from build123d import *

# Parameters (mm, degrees)
SKETCH1_R           = 15
SKETCH1_R_2         = 1.5
SKETCH1_R_3         = 4.7
BOSS_EXTRUDE2_DEPTH = 10
SKETCH2_R           = 1.5
CUT_EXTRUDE1_DEPTH  = 35


with BuildPart() as part:
    # Sketch1 → Boss-Extrude2 (new body)
    with BuildSketch(Plane.XY):
        Circle(SKETCH1_R)
        with Locations((0, 10)):
            Circle(SKETCH1_R_2, mode=Mode.SUBTRACT)
        Circle(SKETCH1_R_3, mode=Mode.SUBTRACT)
        with Locations((10, 0)):
            Circle(SKETCH1_R_2, mode=Mode.SUBTRACT)
        with Locations((0, -10)):
            Circle(SKETCH1_R_2, mode=Mode.SUBTRACT)
        with Locations((-10, 0)):
            Circle(SKETCH1_R_2, mode=Mode.SUBTRACT)
    extrude(amount=BOSS_EXTRUDE2_DEPTH)

    # Sketch2 → Cut-Extrude1 (cut)
    with BuildSketch(Plane(origin=(0, 0, 0), x_dir=(1, 0, 0), z_dir=(0, 1, 0))):
        with Locations(Location((0, -5, 0), (0, 0, 270))):
            Circle(SKETCH2_R)
    extrude(amount=-CUT_EXTRUDE1_DEPTH, mode=Mode.SUBTRACT)


solid = part.part
Check sheet for the modelled part. Datum: model origin and axes. Units: mm. A direction names the side the tool comes from. Round coordinates to 2 decimals unless told otherwise and drop trailing zeros. Order: outer loops, then holes, each group sorted by start corner. A loop starts at its lowest first (then second) coordinate and runs counter-clockwise, first axis right, second up. Notation, with made-up numbers: M 43.5,34 L 95.5,34 A31 ccw 95.5,66 Z; hole C 79,50.25 d9. An arc over 180 degrees is marked long. One line per item, written item: value. Start each with the question number.
1. Scan lines: line 1 along Y through (x, z) = (0, 3); line 2 along X through (y, z) = (-0.5, 5.75). Record each from-to range of solid material in increasing order.
2. Gauge pin test, flat ends, axial feed: P1, Ø2.5, axis at x = 0, y = -10, coming from the -Z side; P2, Ø2, axis at y = -2, z = 9, coming from the -X side; P3, Ø2.5, axis at x = 0, z = 5, coming from the -Y side; P4, Ø1.5, axis at x = 3, z = 1, coming from the -Y side. Record the tip position at first contact, or that the pin passes through.
3. Section check C-C on z = 1. Enter the section's corners in (x, y), and give its area (3 significant figures).
4. Section check A-A on x = 0. Enter the section's corners in (y, z), and give its area (3 significant figures).
5. Section check D-D on x = 10. Enter the section's corners in (y, z), and give its area (3 significant figures).
6. Access from +Z, -Z, +X, -X, +Y, -Y to the whole of each face (thin tool, end or side, straight path). Record for faces 4 (the cylindrical face through (-0.575, -6.572, 6.386)), 5 (the cylindrical face through (1.386, -10.575, 8.021)).
7. Section check B-B on y = 0. Enter the section's corners in (x, z).
8. Release check for a two-part mould opening along Z. For faces 1 (the flat face through (3, 4, 10)), 2 (the cylindrical face through (8.5, 0.07, 4.93)), 3 (the cylindrical face through (0.07, -13.02, 3.5)) record: released by +Z, released by -Z, zero draft, split by the parting line, or undercut.
Results found:
1. line 1: -15 to -11.5, -8.5 to -4.7, 4.7 to 8.5, 11.5 to 15
1. line 2: -14.99 to -11.41, -8.59 to -4.67, 4.67 to 8.59, 11.41 to 14.99
2. P1: through
2. P2: x = -14.97
2. P3: y = 4.53
2. P4: y = -14.83
3. outline: C 0,0 d30; hole C -10,0 d3; hole C 0,0 d9.4; hole C 0,-10 d3; hole C 0,10 d3; hole C 10,0 d3
3. area: 609 mm^2
4. outline: M -15,0 L -11.5,0 L -11.5,3.5 L -15,3.5 Z; M -15,6.5 L -11.5,6.5 L -11.5,10 L -15,10 Z; M -8.5,0 L -4.7,0 L -4.7,3.5 L -8.5,3.5 Z; M -8.5,6.5 L -4.7,6.5 L -4.7,10 L -8.5,10 Z; M 4.7,0 L 8.5,0 L 8.5,10 L 4.7,10 Z; M 11.5,0 L 15,0 L 15,10 L 11.5,10 Z
4. area: 124 mm^2
5. outline: M -11.18,0 L -1.5,0 L -1.5,10 L -11.18,10 Z; M 1.5,0 L 11.18,0 L 11.18,10 L 1.5,10 Z
5. area: 194 mm^2
6. face 4: -Y
6. face 5: +Z, -Z
7. outline: M -15,0 L -11.5,0 L -11.5,10 L -15,10 Z; M -8.5,0 L -4.7,0 L -4.7,10 L -8.5,10 Z; M 4.7,0 L 8.5,0 L 8.5,10 L 4.7,10 Z; M 11.5,0 L 15,0 L 15,10 L 11.5,10 Z
8. face 1: released by +Z
8. face 2: zero draft
8. face 3: undercut
